from build123d import *

# Parameters (mm, degrees)
SKETCH_1_W                = 20
SKETCH_1_H                = 30
EXTRUDE_1_DEPTH           = 150
SKETCH_2_W                = 18
SKETCH_2_H                = 28
CUT_EXTRUDE_1_DEPTH       = 301
SKETCH_3_R                = 1.525
CUT_EXTRUDE_2_DEPTH       = 21
SKETCH_4_R                = 1.525
CUT_EXTRUDE_3_DEPTH       = 31
SKETCH_5_R                = 1.525
CUT_EXTRUDE_4_DEPTH       = 31
SKETCH_6_OUTSIDE_W        = 92.432
SKETCH_6_OUTSIDE_H        = 362.432
SKETCH_6_OUTSIDE_W_2      = 30
SKETCH_6_OUTSIDE_H_2      = 300
SKETCH_6_OUTSIDE_R        = 1.525
CUT_EXTRUDE_6_DEPTH       = 21
CUT_EXTRUDE_8_REACH       = 32
SKETCH_9_R                = 1.525
SKETCH_10_R               = 1.525
CUT_EXTRUDE_9_DEPTH       = 1
CUT_EXTRUDE_9_DEPTH_BACK  = 21
SKETCH_11_R               = 1.525
CUT_EXTRUDE_10_DEPTH      = 20
CUT_EXTRUDE_10_DEPTH_BACK = 2


with BuildPart() as part:
    # 草图1 → 凸台-拉伸1 (new body, symmetric)
    with BuildSketch(Plane(origin=(0, 0, 0), x_dir=(1, 0, 0), z_dir=(0, 1, 0))):
        Rectangle(SKETCH_1_W, SKETCH_1_H)
    extrude(amount=EXTRUDE_1_DEPTH, both=True)

    # 草图2 → 切除-拉伸1 (cut, through all)
    with BuildSketch(Plane(origin=(0, 150, 0), x_dir=(1, 0, 0), z_dir=(0, 1, 0))):
        Rectangle(SKETCH_2_W, SKETCH_2_H)
    extrude(amount=-CUT_EXTRUDE_1_DEPTH, mode=Mode.SUBTRACT)

    # 草图3 → 切除-拉伸2 (cut, through all)
    with BuildSketch(Plane(origin=(10, 0, 0), x_dir=(0, 0, -1), z_dir=(1, 0, 0))):
        with Locations((-1, -146)):
            Circle(SKETCH_3_R)
    extrude(amount=-CUT_EXTRUDE_2_DEPTH, mode=Mode.SUBTRACT)

    # 草图4 → 切除-拉伸3 (cut, through all)
    with BuildSketch(Plane.XY.offset(15)):
        with Locations((0, -146)):
            Circle(SKETCH_4_R)
    extrude(amount=-CUT_EXTRUDE_3_DEPTH, mode=Mode.SUBTRACT)

    # 草图5 → 切除-拉伸4 (cut, through all)
    with BuildSketch(Plane.XY.offset(15)):
        with Locations((0, -136)):
            Circle(SKETCH_5_R)
    extrude(amount=-CUT_EXTRUDE_4_DEPTH, mode=Mode.SUBTRACT)

    # 草图6 outside → 切除-拉伸6 (cut, through all)
    with BuildSketch(Plane(origin=(10, 0, 0), x_dir=(0, 0, -1), z_dir=(1, 0, 0))):
        Rectangle(SKETCH_6_OUTSIDE_W, SKETCH_6_OUTSIDE_H)
        Rectangle(SKETCH_6_OUTSIDE_W_2, SKETCH_6_OUTSIDE_H_2, mode=Mode.SUBTRACT)
        with Locations((-1, -131)):
            Circle(SKETCH_6_OUTSIDE_R)
    extrude(amount=-CUT_EXTRUDE_6_DEPTH, mode=Mode.SUBTRACT)

    # 草图9 → 切除-拉伸8 (cut, up to next)
    with BuildSketch(Plane.XY.offset(15), mode=Mode.PRIVATE) as cut_extrude_8_sk1:
        with Locations((0, -131.5)):
            Circle(SKETCH_9_R)
    cut_extrude_8_tool1 = extrude(cut_extrude_8_sk1.sketch, amount=-CUT_EXTRUDE_8_REACH, mode=Mode.PRIVATE) & part.part
    add(cut_extrude_8_tool1.solids().sort_by_distance((0, -131.5, 15))[0], mode=Mode.SUBTRACT)

    # 草图10 → 切除-拉伸9 (cut, two sides)
    with BuildSketch(Plane(origin=(10, 0, 0), x_dir=(0, 0, -1), z_dir=(1, 0, 0))) as cut_extrude_9_sk:
        with Locations((-1, -136.5)):
            Circle(SKETCH_10_R)
    extrude(amount=CUT_EXTRUDE_9_DEPTH, mode=Mode.SUBTRACT)
    extrude(cut_extrude_9_sk.sketch, amount=-CUT_EXTRUDE_9_DEPTH_BACK, mode=Mode.SUBTRACT)

    # 草图11 → 切除-拉伸10 (cut, two sides)
    with BuildSketch(Plane.ZY.offset(-9)) as cut_extrude_10_sk:
        with Locations((9, 147)):
            Circle(SKETCH_11_R)
        with Locations((-3.5, 147)):
            Circle(SKETCH_11_R)
    extrude(amount=CUT_EXTRUDE_10_DEPTH, mode=Mode.SUBTRACT)
    extrude(cut_extrude_10_sk.sketch, amount=-CUT_EXTRUDE_10_DEPTH_BACK, mode=Mode.SUBTRACT)


solid = part.part
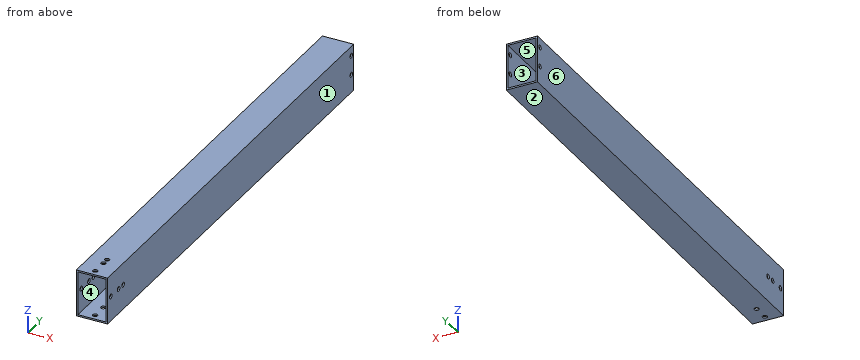
Work out the finished part from the listing and answer in its coordinate system (mm). Face numbers are marked on the shaded views. A direction names the side the tool comes from. Coordinates: 2 decimals unless noted, no trailing zeros. Write each loop counter-clockwise with the first axis right and the second up, starting at its lowest first coordinate (ties: lowest second). Pieces come first, ordered by that corner, then holes.
1. The part is cut by section A-A, the plane y = 107. Write down the section's boundary in (x, z).
Results list:
outline: (-10, -15) - (10, -15) - (10, 15) - (-10, 15) - close; hole (-9, -14) - (9, -14) - (9, 14) - (-9, 14) - close
2. Consider line 1 along Y through (x, z) = (0, 14.75) (3 decimals); line 2 along Y through (x, z) = (-9.6, 1) (3 decimals); line 3 along Z through (x, y) = (9.7, 147) (3 decimals). Determine where each line is inside the solid, lowest interval first.
Results list:
line 1: y = -150 to -147.525, -144.475 to -137.525, -134.475 to -133.025, -129.975 to 150
line 2: y = -150 to -147.525, -144.475 to -138.025, -134.975 to -132.525, -129.475 to 150
line 3: z = -15 to -5.025, -1.975 to 7.475, 10.525 to 15
3. For the marked faces 5 and 6, determine the directions among +Z, -Z, +X, -X, +Y, -Y from which every point of the face is accessible in a straight line to the end or side of a thin tool.
Results list:
face 5: +Y, -Y
face 6: +Z, -Z, -X, +Y, -Y
4. A flat-ended cylindrical pin translates along its axis: pin 1 (2.5 mm diameter, centred on y = -146, z = 1, fed in from -X). Find the tip coordinate at first contact, or state that the pin passes through.
Results list:
pin 1: passes through
5. For a pull along X with two mould halves and no side action, classify the marked faces 1, 2, 3 and 4 as +X half, -X half, draft (parallel to the pull), parting line (faces both ways), or undercut.
Results list:
face 1: +X half
face 2: draft
face 3: undercut
face 4: undercut
